Work out the finished part from the listing and answer in its coordinate system (mm). A direction names the side the tool comes from. Give positions to 0.01 mm unless a question says otherwise; leave off trailing zeros. Order: outer loops, then holes, each group sorted by start corner. A loop starts at its lowest first (then second) coordinate and runs counter-clockwise, first axis right, second up.
```python
from build123d import *

# Parameters (mm, degrees)
SKETCH1_W           = 200
SKETCH1_H           = 110
BOSS_EXTRUDE1_DEPTH = 20
FILLET2_R           = 30
SKETCH2_R           = 5
CUT_EXTRUDE1_DEPTH  = 24
CHAMFER1_SIZE       = 5
BOSS_EXTRUDE2_DEPTH = 1
CUT_EXTRUDE2_DEPTH  = 5
CHAMFER2_SIZE       = 1
CHAMFER3_SIZE       = 2
CHAMFER4_SIZE       = 3


with BuildPart() as part:
    # Sketch1 → Boss-Extrude1 (new body)
    with BuildSketch(Plane(origin=(0, 0, 0), x_dir=(1, 0, 0), z_dir=(0, 1, 0))):
        with Locations((22.74566474, -0.63583815)):
            Rectangle(SKETCH1_W, SKETCH1_H)
    extrude(amount=BOSS_EXTRUDE1_DEPTH)

    # Fillet2
    fillet2_edges = [part.edges().sort_by_distance(p)[0] for p in [
        (122.74566474, 10, -54.36416185),
        (122.74566474, 10, 55.63583815),
    ]]
    fillet(fillet2_edges, radius=FILLET2_R)

    # Sketch4 → section 0 of loft1
    with BuildSketch(Plane(origin=(0, -60, 0), x_dir=(-1, 0, 0), z_dir=(0, -1, 0)), mode=Mode.PRIVATE) as loft1_s0:
        with BuildLine():
            Line((-122.74566474, 24.36416185), (-122.74566474, -25.63583815))
            ThreePointArc((-122.74566474, -25.63583815), (-113.958868175, -46.849041586), (-92.74566474, -55.63583815))
            Line((-92.74566474, -55.63583815), (77.25433526, -55.63583815))
            Line((77.25433526, -55.63583815), (77.25433526, 54.36416185))
            Line((77.25433526, 54.36416185), (-92.74566474, 54.36416185))
            ThreePointArc((-92.74566474, 54.36416185), (-113.958868175, 45.577365285), (-122.74566474, 24.36416185))
        make_face()
    # loft up to a face of the part (loft1)
    loft([loft1_s0.sketch, part.faces().sort_by_distance((21.078212912, 0, 0.63583815))[0]])

    # Sketch2 → Cut-Extrude1 (cut)
    with BuildSketch(Plane(origin=(0, 20, 0), x_dir=(1, 0, 0), z_dir=(0, 1, 0))):
        with Locations((72.74566474, -3.505923633)):
            Circle(SKETCH2_R)
    extrude(amount=-CUT_EXTRUDE1_DEPTH, mode=Mode.SUBTRACT)

    # Chamfer1
    chamfer1_edges = [part.edges().sort_by_distance(p)[0] for p in [
        (113.958868175, 20, 46.849041586),
        (7.74566474, 20, 55.63583815),
        (-77.25433526, 20, 0.63583815),
        (7.74566474, 20, -54.36416185),
        (113.958868175, 20, -45.577365285),
        (122.74566474, 20, 0.63583815),
    ]]
    chamfer(chamfer1_edges, length=CHAMFER1_SIZE)

    # Sketch5 → Boss-Extrude2 (add)
    with BuildSketch(Plane.XY.offset(55.63583815)):
        with BuildLine():
            ThreePointArc((-68.75433526, -13.5), (-68.168548822, -12.085786438), (-66.75433526, -11.5))
            Line((-66.75433526, -11.5), (-0.75433526, -11.5))
            ThreePointArc((-0.75433526, -11.5), (0.659878302, -12.085786438), (1.24566474, -13.5))
            Line((1.24566474, -13.5), (1.24566474, -49.5))
            ThreePointArc((1.24566474, -49.5), (0.659878302, -50.914213562), (-0.75433526, -51.5))
            Line((-0.75433526, -51.5), (-66.75433526, -51.5))
            ThreePointArc((-66.75433526, -51.5), (-68.168548822, -50.914213562), (-68.75433526, -49.5))
            Line((-68.75433526, -49.5), (-68.75433526, -13.5))
        make_face()
    extrude(amount=BOSS_EXTRUDE2_DEPTH)

    # Sketch6 → Cut-Extrude2 (cut)
    with BuildSketch(Plane.ZY.offset(77.25433526)):
        with BuildLine():
            Line((40.63583815, 5), (-39.36416185, 5))
            ThreePointArc((-39.36416185, 5), (-42.899695756, 3.535533906), (-44.36416185, 0))
            Line((-44.36416185, 0), (-44.36416185, -50))
            Line((-44.36416185, -50), (45.63583815, -50))
            Line((45.63583815, -50), (45.63583815, 0))
            ThreePointArc((45.63583815, 0), (44.171372056, 3.535533906), (40.63583815, 5))
        make_face()
    extrude(amount=-CUT_EXTRUDE2_DEPTH, mode=Mode.SUBTRACT)

    # Chamfer2
    chamfer2_edges = [part.edges().sort_by_distance(p)[0] for p in [
        (-77.25433526, 3.535533906, 44.171372056),
        (-77.25433526, 5, 0.63583815),
        (-77.25433526, 3.535533906, -42.899695756),
        (-77.25433526, -25, -44.36416185),
        (-77.25433526, -50, 0.63583815),
        (-77.25433526, -25, 45.63583815),
    ]]
    chamfer(chamfer2_edges, length=CHAMFER2_SIZE)

    # Chamfer3
    chamfer3_edges = [part.edges().sort_by_distance(p)[0] for p in [
        (67.74566474, 20, 3.505923633),
    ]]
    chamfer(chamfer3_edges, length=CHAMFER3_SIZE)

    # Chamfer4
    chamfer4_edges = [part.edges().sort_by_distance(p)[0] for p in [
        (-77.25433526, -22.5, 55.63583815),
        (-77.25433526, -22.5, 55.63583815),
        (-77.25433526, -22.5, -54.36416185),
        (-77.25433526, -22.5, -54.36416185),
    ]]
    chamfer(chamfer4_edges, length=CHAMFER4_SIZE)


solid = part.part
```
1. Straight lines are drawn through the part: probe 1 along Z at (x, y) = (49.5, 8.5); probe 2 along X at (y, z) = (-41, 23); probe 3 along X at (y, z) = (3, 6). For each, find the intervals that lie inside material, in ascending order.
Findings below:
probe 1: z = -54.36 to 55.64
probe 2: x = -72.25 to 122.75
probe 3: x = -72.25 to 68.41, 77.08 to 122.75
2. The mould has two halves that part along X. Classify faces 3 (the face through (21, -60, 1)), 4 (the face through (-76.525, 3.686, 44.404)), 5 (the face through (77.364, 7.154, 5.421)): pulls with the +X half, pulls with the -X half, needs draft (parallel to the pull), parting line crosses it, or undercut.
Findings below:
face 3: needs draft
face 4: pulls with the -X half
face 5: undercut
3. The part is cut by section A-A (y = -18). Write down the section's boundary in (x, z).
Findings below:
outline: (-77.25, -51.36) - (-74.25, -54.36) - (92.75, -54.36) arc R30 ccw to (122.75, -24.36) - (122.75, 25.64) arc R30 ccw to (92.75, 55.64) - (1.25, 55.64) - (1.25, 56.64) - (-68.75, 56.64) - (-68.75, 55.64) - (-74.25, 55.64) - (-77.25, 52.64) - (-77.25, 46.64) - (-76.25, 45.64) - (-72.25, 45.64) - (-72.25, -44.36) - (-76.25, -44.36) - (-77.25, -45.36) - close
4. Given P1, Ø3, axis at x = 71, z = 5, coming from the +Y side; P2, Ø5, axis at x = 75.5, y = -39.5, coming from the +Z side; P3, Ø0.8, axis at x = -30, z = 56, coming from the +Y side; P4, Ø12, axis at y = -50.5, z = 12.5, coming from the -X side, each flat-ended and moving along its own axis, determine where each tip first touches the part or whether it passes through.
Findings below:
P1: stops at y = -4
P2: stops at z = 55.64
P3: stops at y = 15.04
P4: stops at x = -77.25
5. The part is cut by section B-B (z = 23). Write down the section's boundary in (x, y), then the cut area to 3 significant figures.
Findings below:
outline: (-77.25, -60) - (122.75, -60) - (122.75, 15) - (117.75, 20) - (-72.25, 20) - (-77.25, 15) - (-77.25, 6) - (-76.25, 5) - (-72.25, 5) - (-72.25, -50) - (-76.25, -50) - (-77.25, -51) - close
area: 15,700 mm2
6. The part is cut by section C-C (y = -8). Write down the section's boundary in (x, z), then the cut area to 3 significant figures.
Findings below:
outline: (-77.25, -51.36) - (-74.25, -54.36) - (92.75, -54.36) arc R30 ccw to (122.75, -24.36) - (122.75, 25.64) arc R30 ccw to (92.75, 55.64) - (-74.25, 55.64) - (-77.25, 52.64) - (-77.25, 46.64) - (-76.25, 45.64) - (-72.25, 45.64) - (-72.25, -44.36) - (-76.25, -44.36) - (-77.25, -45.36) - close
area: 21,200 mm2
7. Which of the six approach directions +Z, -Z, +X, -X, +Y, -Y give full straight-line access (tool end or side, diameter ignored) to faces 1 (the face through (8, -22, -54.364)), 2 (the face through (-74, 5, 1))?
Findings below:
face 1: -Z, +X, -X, +Y, -Y
face 2: -X
